```python
from build123d import *

# Parameters (mm, degrees)
BOSS_EXTRUDE1_DEPTH  = 1.72
CUT_EXTRUDE1_DEPTH   = 1.72
SKETCH6_W            = 5.52
SKETCH6_H            = 11.86
SKETCH6_W_2          = 10.85
SKETCH6_H_2          = 5.52
SWITCHES_DEPTH       = 6.28
SKETCH7_W            = 10.8
SKETCH7_H            = 6.18
SCROLLWHEEL_DEPTH    = 16.82
SKETCH8_W            = 20.3
SKETCH8_H            = 12.86
CHIP_DEPTH           = 2.52
SKETCH9_W            = 12.02
SKETCH9_H            = 4.82
USB_CONNECTION_DEPTH = 6.34
SKETCH10_W           = 12.47
SKETCH10_H           = 8.02
LASER_DEPTH          = 6.54


with BuildPart() as part:
    # Sketch1 → Boss-Extrude1 (new body)
    with BuildSketch(Plane(origin=(0, 0, 0), x_dir=(1, 0, 0), z_dir=(0, 1, 0))):
        Polygon((46.12, 45.94), (71.12, 45.94), (71.12, 4.17), (46.12, 4.17), (46.12, 0), (0, 0), (0, 50.09), (46.12, 50.09), align=None)
    extrude(amount=-BOSS_EXTRUDE1_DEPTH)

    # Sketch2 → Cut-Extrude1 (cut)
    with BuildSketch(Plane(origin=(0, 0, 0), x_dir=(1, 0, 0), z_dir=(0, 1, 0))):
        Polygon((65.72, 32.46), (54.12, 32.46), (54.12, 29.58), (52.14, 29.58), (52.14, 19.94), (54.12, 19.94), (54.12, 17.62), (65.72, 17.62), (65.72, 19.94), (68.16, 19.94), (68.16, 29.58), (65.72, 29.58), align=None)
        Polygon((17.483002282, 20.9), (17.483002282, 19.69), (14.863002282, 19.69), (14.863002282, 20.9), (10.663002282, 20.9), (10.663002282, 29.4), (14.863002282, 29.4), (14.863002282, 30.69), (17.483002282, 30.69), (17.483002282, 29.4), (44.54, 29.4), (44.54, 20.9), align=None)
    extrude(amount=-CUT_EXTRUDE1_DEPTH, mode=Mode.SUBTRACT)

    # Sketch6 → switches (add)
    with BuildSketch(Plane(origin=(0, 0, 0), x_dir=(1, 0, 0), z_dir=(0, 1, 0))):
        with Locations((68.36, 10.1)):
            Rectangle(SKETCH6_W, SKETCH6_H)
        with Locations((61.6, 10.1)):
            Rectangle(SKETCH6_W, SKETCH6_H)
        with Locations((65.695, 43.18)):
            Rectangle(SKETCH6_W_2, SKETCH6_H_2)
    extrude(amount=SWITCHES_DEPTH)

    # Sketch7 → scrollWheel (add)
    with BuildSketch(Plane(origin=(0, 0, 0), x_dir=(1, 0, 0), z_dir=(0, 1, 0))):
        with Locations((60.67, 36.83)):
            Rectangle(SKETCH7_W, SKETCH7_H)
    extrude(amount=SCROLLWHEEL_DEPTH)

    # Sketch8 → chip (add)
    with BuildSketch(Plane(origin=(0, 0, 0), x_dir=(1, 0, 0), z_dir=(0, 1, 0))):
        with Locations((34.97, 25.26)):
            Rectangle(SKETCH8_W, SKETCH8_H)
    extrude(amount=CHIP_DEPTH)

    # Sketch9 → USB Connection (add)
    with BuildSketch(Plane(origin=(0, 0, 0), x_dir=(1, 0, 0), z_dir=(0, 1, 0))):
        with Locations((29.14, 45.94)):
            Rectangle(SKETCH9_W, SKETCH9_H)
    extrude(amount=USB_CONNECTION_DEPTH)

    # Sketch10 → laser (add)
    with BuildSketch(Plane(origin=(0, 0, 0), x_dir=(1, 0, 0), z_dir=(0, 1, 0))):
        with Locations((10.755, 25.01)):
            Rectangle(SKETCH10_W, SKETCH10_H)
    extrude(amount=LASER_DEPTH)


solid = part.part
```
The model under review builds one solid part; all positions refer to its coordinate system, in mm. A direction names the side the tool comes from. Round coordinates to 2 decimals unless told otherwise and drop trailing zeros. Write each loop counter-clockwise with the first axis right and the second up, starting at its lowest first coordinate (ties: lowest second). Pieces come first, ordered by that corner, then holes.
(1) We need section A-A on z = -26. Give the boundary of the cut face in (x, y), and give its area (3 significant figures).
(2) Insertion check: pin 1 (0.5 mm diameter, centred on y = -1, z = -23, fed in from -X); pin 2 (1.5 mm diameter, centred on x = 24, y = 7, fed in from -Z); pin 3 (7 mm diameter, centred on x = 68, y = 2.5, fed in from +Z); pin 4 (3 mm diameter, centred on x = 63, z = -9, fed in from +Y). Each pin has a flat end and moves straight along its axis. Give the tip position at first contact, or say it passes through.
(3) Mouldability with a two-part tool opening along Z and no side actions: class faces 4 (the flat face through (35, 1, -18.83)), 5 (the flat face through (14, 0, -25)), 6 (the flat face through (16.99, 3, -25)), 7 (the flat face through (65.72, -1, -31)) as +Z half, -Z half, draft (parallel to the pull), parting line (faces both ways), or undercut.
(4) Machinability: for faces 1 (the flat face through (60.27, 3, -43)), 2 (the flat face through (46.12, -1, -2)), 3 (the flat face through (11, 3, -29.02)), which of the approach directions +Z, -Z, +X, -X, +Y, -Y give a long, thin tool a straight path to every point of the face, cutting with its end or side? Answer none if there is none.
(5) We need section D-D on x = 42.5. Give the boundary of the cut face in (y, z), and give its area (3 significant figures).
(6) We need section C-C on y = 4. Give the boundary of the cut face in (x, z).
(7) Wall thickness on L1, parallel to Z at x = 65, y = -0.25; L2, parallel to Z at x = 64.5, y = 2.75; L3, parallel to Y at x = 43, z = -39.5: over which ranges is each line inside the solid? List them lowest first.
(8) We need section B-B on x = 61.5. Give the boundary of the cut face in (y, z), and give its area (3 significant figures).
Findings below:
1. outline: (0, -1.72) - (10.66, -1.72) - (10.66, 0) - (16.99, 0) - (16.99, 6.54) - (4.52, 6.54) - (4.52, 0) - (0, 0) - close; (24.82, 0) - (44.54, 0) - (44.54, -1.72) - (52.14, -1.72) - (52.14, 0) - (45.12, 0) - (45.12, 2.52) - (24.82, 2.52) - close; (68.16, -1.72) - (71.12, -1.72) - (71.12, 0) - (68.16, 0) - close
1. area: 169 mm2
2. pin 1: stops at x = 0
2. pin 2: stops at z = -48.35
2. pin 3: stops at z = -4.17
2. pin 4: stops at y = 6.28
3. face 4: +Z half
3. face 5: undercut
3. face 6: draft
3. face 7: undercut
4. face 1: -Z, +Y
4. face 2: +Z, +X, +Y, -Y
4. face 3: -Z, -X, +Y
5. outline: (-1.72, -50.09) - (0, -50.09) - (0, -31.69) - (2.52, -31.69) - (2.52, -18.83) - (0, -18.83) - (0, 0) - (-1.72, 0) - (-1.72, -20.9) - (0, -20.9) - (0, -29.4) - (-1.72, -29.4) - close
5. area: 104 mm2
6. outline: (4.52, -29.02) - (16.99, -29.02) - (16.99, -21) - (4.52, -21) - close; (23.13, -48.35) - (35.15, -48.35) - (35.15, -43.53) - (23.13, -43.53) - close; (55.27, -39.92) - (66.07, -39.92) - (66.07, -33.74) - (55.27, -33.74) - close; (58.84, -16.03) - (64.36, -16.03) - (64.36, -4.17) - (58.84, -4.17) - close; (60.27, -45.94) - (71.12, -45.94) - (71.12, -40.42) - (60.27, -40.42) - close; (65.6, -16.03) - (71.12, -16.03) - (71.12, -4.17) - (65.6, -4.17) - close
7. L1: z = -45.94 to -32.46, -17.62 to -4.17
7. L2: z = -45.94 to -40.42, -39.92 to -33.74
7. L3: y = -1.72 to 0
8. outline: (-1.72, -45.94) - (6.28, -45.94) - (6.28, -40.42) - (0, -40.42) - (0, -39.92) - (16.82, -39.92) - (16.82, -33.74) - (0, -33.74) - (0, -32.46) - (-1.72, -32.46) - close; (-1.72, -17.62) - (0, -17.62) - (0, -16.03) - (6.28, -16.03) - (6.28, -4.17) - (-1.72, -4.17) - close
8. area: 259 mm2
